Check sheet for the modelled part. Datum: model origin and axes. Units: mm. A direction names the side the tool comes from. Coordinates: 2 decimals unless noted, no trailing zeros. Write each loop counter-clockwise with the first axis right and the second up, starting at its lowest first coordinate (ties: lowest second). Pieces come first, ordered by that corner, then holes. Notation, with made-up numbers: (40, 69) - (94, 69) arc R15 ccw to (94, 96) - close; hole circle Ø4 at (37, 45.5). An arc over 180 degrees is marked (long way). Use one line per item in the form item = value. Start each with the question number.
1. Draft check along X on faces 1 (the face through (-144.99, 0.99, 2.96)), 2 (the face through (105, 0, 4)), 3 (the face through (-2, 11, 6)). Enter one of: +X half, -X half, draft (parallel to the pull), parting line (faces both ways), or undercut.
2. Scan lines: line 1 along Y through (x, z) = (-29, 3.7); line 2 along Z through (x, y) = (-15, 3.5); line 3 along X through (y, z) = (-20, 3.3). Record each from-to range of solid material in increasing order.
3. Go/stop test with flat-tipped pins: pin 1 Ø1 at (y, z) = (-35.5, 2) entering from -X; pin 2 Ø1 at (y, z) = (20, 1) entering from +X; pin 3 Ø5 at (x, y) = (7.5, 0) entering from +Z; pin 4 Ø5 at (x, y) = (-38.5, -16.5) entering from -Z. Record where each tip stops, or that it passes through.
4. Cross-section at A-A on z = 4.3. Record the boundary of the cut face in (x, y).
5. Tool access check on faces 4 (the face through (-1, -45, 3)), 5 (the face through (-105, 0, 4)). Record the directions out of +Z, -Z, +X, -X, +Y, -Y that give a thin tool (end or side, any length) a straight path to the whole face; none if there is none.
6. Cross-section at D-D on y = -28.5. Record the boundary of the cut face in (x, z).
7. Cross-section at C-C on y = 0. Record the boundary of the cut face in (x, z), then the cut area to 3 significant figures.
8. Cross-section at B-B on x = 14.5. Record the boundary of the cut face in (y, z).
```python
from build123d import *

# Parameters (mm, degrees)
PAD_DEPTH    = 3
PAD001_DEPTH = 3


with BuildPart() as part:
    # Sketch → Pad (new body)
    with BuildSketch(Plane.XY):
        with BuildLine():
            ThreePointArc((-100, 45), (-145, 0), (-100, -45))
            Line((-100, -45), (100, -45))
            ThreePointArc((100, -45), (145, 0), (100, 45))
            Line((-100, 45), (100, 45))
        make_face()
    extrude(amount=PAD_DEPTH)

    # Sketch001 (on Face6 of Pad) → Pad001 (join)
    with BuildSketch(Plane.XY.offset(3)):
        with BuildLine():
            ThreePointArc((-100, 45), (-145, 0), (-100, -45))
            Line((-100, -45), (100, -45))
            ThreePointArc((100, -45), (145, 0), (100, 45))
            Line((-100, 45), (100, 45))
        make_face()
        with BuildLine():
            ThreePointArc((-100, 5), (-105, 0), (-100, -5))
            Line((-100, -5), (100, -5))
            ThreePointArc((100, -5), (105, 0), (100, 5))
            Line((-100, 5), (100, 5))
        make_face(mode=Mode.SUBTRACT)
    extrude(amount=PAD001_DEPTH)


solid = part.part
```
Final values:
q1.face_1 = -X half
q1.face_2 = undercut
q1.face_3 = draft
q2.line_1 = -45 to -5, 5 to 45
q2.line_2 = 0 to 3
q2.line_3 = -140.31 to 140.31
q3.pin_1 = -128.28
q3.pin_2 = 140.56
q3.pin_3 = 3
q3.pin_4 = 0
q4.outline = (-100, -45) - (100, -45) arc R45 ccw to (100, 45) - (-100, 45) arc R45 ccw to start; hole (-100, -5) - (100, -5) arc R5 ccw to (100, 5) - (-100, 5) arc R5 ccw to start
q5.face_4 = +Z, -Z, +X, -X, -Y
q5.face_5 = +Z
q6.outline = (-134.82, 0) - (134.82, 0) - (134.82, 6) - (-134.82, 6) - close
q7.outline = (-145, 0) - (145, 0) - (145, 6) - (105, 6) - (105, 3) - (-105, 3) - (-105, 6) - (-145, 6) - close
q7.area = 1,110 mm²
q8.outline = (-45, 0) - (45, 0) - (45, 6) - (5, 6) - (5, 3) - (-5, 3) - (-5, 6) - (-45, 6) - close
